Source: CAD feature listing. Evaluate the final solid. Frame: model axes, mm. A direction names the side the tool comes from. Give positions to 0.01 mm unless a question says otherwise; leave off trailing zeros. Write each loop counter-clockwise with the first axis right and the second up, starting at its lowest first coordinate (ties: lowest second). Pieces come first, ordered by that corner, then holes. Notation, with made-up numbers: (-34.75, 66.25) -> (-18.75, 66.25) arc R15 ccw to (-18.75, 72.25) -> close; hole circle Ø5 at (-2, -22.5). An arc over 180 degrees is marked (long way). Answer as a JSON object with one key per item and string values. Group by question number.
Item 1: First-contact query: pin 1 Ø11 at (x, z) = (10, 59.5) entering from +Y; pin 2 Ø1 at (y, z) = (119, 23.5) entering from -X; pin 3 Ø6 at (x, z) = (9, 47.5) entering from -Y; pin 4 Ø4 at (x, y) = (7.5, 97.5) entering from +Z. Flat tips, straight axial feed; report the tip coordinate or a pass-through.
Item 2: Section query D-D on y = 138. Return the cut outline in (x, z).
Item 3: Access query for faces 4 (the face through (13, 149, 48)), 5 (the face through (12.675, 44.274, 59.609)). Directions: +Z, -Z, +X, -X, +Y, -Y. A direction counts if a zero-diameter tool reaches every point of the face in a straight line with its end or side. Return the directions, or none.
Item 4: Section query A-A on y = 65. Return the cut outline in (x, z), plus the area to 4 significant figures.
Item 5: Pull-direction query (Y, two-part tool) for faces 1 (the face through (12, 20, 50)), 2 (the face through (12.325, 28.613, 9.129)), 3 (the face through (12, 74, 0)); classes: pulls with the +Y half, pulls with the -Y half, needs draft (parallel to the pull), parting line crosses it, or undercut.
Item 6: Section query B-B on x = 23. Return the cut outline in (y, z), plus the area to 3 significant figures.
Item 7: Ray query, probe 1 along Z at (x, y) = (19.25, 25); probe 2 along Y at (x, z) = (16, 10); probe 3 along Z at (x, y) = (8, 110). Return the intervals inside material, ascending. Write a range as from..to.
Item 8: Section query C-C on y = 110. Return the cut outline in (x, z), plus the area to 3 significant figures.
from build123d import *

# Parameters (mm, degrees)
F0_R     = 3.787682
F1_DEPTH = 25
F2_R     = 5
F3_R     = 5


with BuildPart() as f1:
    # F0 (on Right) → F1 (new body)
    with BuildSketch(Plane.YZ):
        Polygon((0, 30), (0, 0), (150, 0), (150, 50), (90, 50), (90, 70), (40, 70), align=None)
        with Locations((25, 7.99161)):
            Circle(F0_R, mode=Mode.SUBTRACT)
        with Locations((110, 7.99161)):
            Circle(F0_R, mode=Mode.SUBTRACT)
        Polygon((44.142136, 60), (80, 60), (80, 35), (19.142136, 35), align=None, mode=Mode.SUBTRACT)
    extrude(amount=F1_DEPTH)

    # F2
    f2_edges = [f1.edges().sort_by_distance(p)[0] for p in [
        (12.5, 90, 70),
        (12.5, 90, 50),
        (12.5, 150, 50),
        (12.5, 150, 0),
        (12.5, 40, 70),
        (12.5, 0, 30),
        (12.5, 0, 0),
    ]]
    fillet(f2_edges, radius=F2_R)

    # F3
    f3_edges = [f1.edges().sort_by_distance(p)[0] for p in [
        (12.5, 19.142136, 35),
        (12.5, 80, 60),
        (12.5, 44.142136, 60),
        (12.5, 80, 35),
    ]]
    fillet(f3_edges, radius=F3_R)


solid = f1.part
Worked answers:
{
 "1": {"pin 1": "y = 90.1", "pin 2": "x = 0", "pin 3": "y = 14.5", "pin 4": "z = 50"},
 "2": {"outline": "(0, 0) -> (25, 0) -> (25, 50) -> (0, 50) -> close"},
 "3": {"face 4": "+Z, +X, -X, +Y", "face 5": "+X, -X"},
 "4": {"outline": "(0, 0) -> (25, 0) -> (25, 35) -> (0, 35) -> close; (0, 60) -> (25, 60) -> (25, 70) -> (0, 70) -> close", "area": "1,125 mm^2"},
 "5": {"face 1": "pulls with the -Y half", "face 2": "undercut", "face 3": "needs draft"},
 "6": {"outline": "(0, 5) arc R5 ccw to (5, 0) -> (145, 0) arc R5 ccw to (150, 5) -> (150, 45) arc R5 ccw to (145, 50) -> (95, 50) arc R5 cw to (90, 55) -> (90, 65) arc R5 ccw to (85, 70) -> (42.07, 70) arc R5 ccw to (38.54, 68.54) -> (1.46, 31.46) arc R5 ccw to (0, 27.93) -> close; hole circle Ø7.58 at (25, 7.99); hole (27.68, 43.54) arc R5 ccw to (31.21, 35) -> (75, 35) arc R5 ccw to (80, 40) -> (80, 55) arc R5 ccw to (75, 60) -> (46.21, 60) arc R5 ccw to (42.68, 58.54) -> close; hole circle Ø7.58 at (110, 7.99)", "area": "7,230 mm^2"},
 "7": {"probe 1": "0..4.2, 11.78..55", "probe 2": "0..21.79, 28.21..106.79, 113.21..150", "probe 3": "0..4.2, 11.78..50"},
 "8": {"outline": "(0, 0) -> (25, 0) -> (25, 4.2) -> (0, 4.2) -> close; (0, 11.78) -> (25, 11.78) -> (25, 50) -> (0, 50) -> close", "area": "1,060 mm^2"}
}
